```python
from build123d import *

# Parameters (mm, degrees)
PAD015_DEPTH    = 2.9972
SKETCH022_R     = 1.524
POCKET002_DEPTH = 2.9972
SKETCH023_R     = 1.524
POCKET003_DEPTH = 2.9972


with BuildPart() as part:
    # Sketch018 → Pad015 (new body)
    with BuildSketch(Plane.XY.offset(-90.4748)):
        with BuildLine():
            Line((-60.96, 43.18), (60.96, 43.18))
            ThreePointArc((73.66, 30.48), (69.940256, 39.460256), (60.96, 43.18))
            Line((73.66, 30.48), (73.66, -30.48))
            ThreePointArc((60.96, -43.18), (69.940256, -39.460256), (73.66, -30.48))
            Line((60.96, -43.18), (-60.96, -43.18))
            ThreePointArc((-73.66, -30.48), (-69.940256, -39.460256), (-60.96, -43.18))
            Line((-73.66, -30.48), (-73.66, 30.48))
            ThreePointArc((-60.96, 43.18), (-69.940256, 39.460256), (-73.66, 30.48))
        make_face()
    extrude(amount=-PAD015_DEPTH)

    # Sketch022 → Pocket002 (cut)
    with BuildSketch(Plane(origin=(0, 0, -93.472), x_dir=(1, 0, 0), z_dir=(0, 0, -1))):
        with Locations((-63.5, 33.02)):
            Circle(SKETCH022_R)
        with Locations((-63.5, -33.02)):
            Circle(SKETCH022_R)
        with Locations((63.5, -33.02)):
            Circle(SKETCH022_R)
        with Locations((63.5, 33.02)):
            Circle(SKETCH022_R)
    extrude(amount=-POCKET002_DEPTH, mode=Mode.SUBTRACT)

    # Sketch023 → Pocket003 (cut)
    with BuildSketch(Plane(origin=(0, 0, -93.472), x_dir=(1, 0, 0), z_dir=(0, 0, -1))):
        with Locations((-22.86, 22.86)):
            Circle(SKETCH023_R)
        with Locations((-22.86, -22.86)):
            Circle(SKETCH023_R)
        with Locations((22.86, -22.86)):
            Circle(SKETCH023_R)
        with Locations((22.86, 22.86)):
            Circle(SKETCH023_R)
    extrude(amount=-POCKET003_DEPTH, mode=Mode.SUBTRACT)


solid = part.part
```
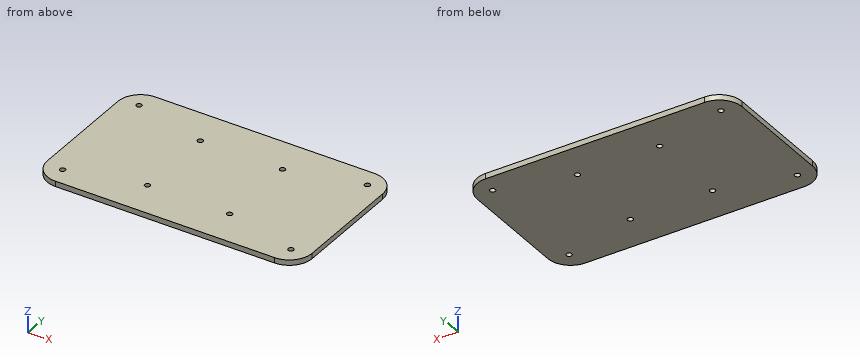
CAD build for the part. Positions are in the model's coordinates, mm. Coordinates: 2 decimals unless noted, no trailing zeros. Loops run counter-clockwise (first coordinate to the right, second up) from the corner with the lowest first, then second, coordinate; pieces in that order, holes last. Notation, with made-up numbers: (7.25, 31) - (52.25, 31) arc R9 ccw to (52.25, 45) - close; hole circle Ø1 at (-19.5, 16). An arc over 180 degrees is marked (long way). Use CSV: the item, a comma, the result in double quotes. Start each with the question number.
Q1. Probe probe 1 along Y at (x, z) = (22.86, -91.2); probe 2 along X at (y, z) = (-22.86, -91.6); probe 3 along X at (y, z) = (33.02, -92.65). List the from-to ranges inside material, lowest first. Write a range as from..to.
Q2. Cut at B-B, the plane y = 22.86. List the corners of the cut face in (x, z).
Q3. Drop flat-ended pins along their axis: P1, Ø5, axis at x = -63.5, y = -33.02, coming from the +Z side; P2, Ø2.5, axis at x = -22.86, y = 22.86, coming from the -Z side (3 decimals). Give the stop position or say it passes through.
Q4. Cut at A-A, the plane x = 22.86. List the corners of the cut face in (y, z).
Q5. Cut at C-C, the plane z = -92. State how many separate pieces and enclosed holes the cut face has, then the cut area to 3 significant figures.
Here are the results:
1,probe 1,"-43.18..-24.38, -21.34..21.34, 24.38..43.18"
1,probe 2,"-73.66..-24.38, -21.34..21.34, 24.38..73.66"
1,probe 3,"-73.4..-65.02, -61.98..61.98, 65.02..73.4"
2,outline,"(-73.66, -93.47) - (-24.38, -93.47) - (-24.38, -90.47) - (-73.66, -90.47) - close; (-21.34, -93.47) - (21.34, -93.47) - (21.34, -90.47) - (-21.34, -90.47) - close; (24.38, -93.47) - (73.66, -93.47) - (73.66, -90.47) - (24.38, -90.47) - close"
3,P1,"z = -90.47"
3,P2,"through"
4,outline,"(-43.18, -93.47) - (-24.38, -93.47) - (-24.38, -90.47) - (-43.18, -90.47) - close; (-21.34, -93.47) - (21.34, -93.47) - (21.34, -90.47) - (-21.34, -90.47) - close; (24.38, -93.47) - (43.18, -93.47) - (43.18, -90.47) - (24.38, -90.47) - close"
5,separate pieces,"1"
5,enclosed holes,"8"
5,area,"12,500 mm2"
